Source: CAD feature listing. Evaluate the final solid. Frame: model axes, mm. Round coordinates to 2 decimals unless told otherwise and drop trailing zeros. Write each loop counter-clockwise with the first axis right and the second up, starting at its lowest first coordinate (ties: lowest second). Pieces come first, ordered by that corner, then holes. Notation, with made-up numbers: M -30.75,16 L -11.75,16 A34 cw -11.75,52 Z; hole C -3,-20.75 d6. An arc over 180 degrees is marked long. Answer in a Markdown table with one row per item.
from build123d import *

# Parameters (mm, degrees)
SKETCH1_R           = 4
SKETCH1_R_2         = 2
BOSS_EXTRUDE1_DEPTH = 5
FILLET1_R           = 1


with BuildPart() as part:
    # Sketch1 → Boss-Extrude1 (new body)
    with BuildSketch(Plane.XY):
        Polygon((0, -20), (8, -40), (12, -40), (20, -20), (20, 0), (0, 0), align=None)
        with Locations((9.984598527, -6.114863432)):
            Circle(SKETCH1_R, mode=Mode.SUBTRACT)
        with Locations((9.984598527, -36.114863432)):
            Circle(SKETCH1_R_2, mode=Mode.SUBTRACT)
    extrude(amount=BOSS_EXTRUDE1_DEPTH)

    # Fillet1
    fillet1_edges = [part.edges().sort_by_distance(p)[0] for p in [
        (10, -40, 5),
        (0, 0, 2.5),
        (20, 0, 2.5),
        (20, -20, 2.5),
        (12, -40, 2.5),
        (8, -40, 2.5),
        (0, -20, 2.5),
        (16, -30, 5),
        (20, -10, 5),
        (10, 0, 5),
        (0, -10, 5),
        (10, 0, 0),
        (20, -10, 0),
        (16, -30, 0),
        (4, -30, 5),
        (10, -40, 0),
        (4, -30, 0),
        (0, -10, 0),
    ]]
    fillet(fillet1_edges, radius=FILLET1_R)


solid = part.part
Q1. Section A-A (y = -7). Return loops of the section in (x, z).
Solutions:
| item | result |
|---|---|
| outline | M 0,1 A1 ccw 1,0 L 6.08,0 L 6.08,5 L 1,5 A1 ccw 0,4 Z; M 13.89,0 L 19,0 A1 ccw 20,1 L 20,4 A1 ccw 19,5 L 13.89,5 Z |
Q2. Pull-direction query (X, two-part tool) for faces 1 (the flat face through (0, -10, 2)), 2 (the cylindrical face through (15.88, -29.53, 0.3)), 3 (the cylindrical face through (5.99, -5.94, 2.46)); classes: pulls with the +X half, pulls with the -X half, needs draft (parallel to the pull), parting line crosses it, or undercut.
Solutions:
| item | result |
|---|---|
| face 1 | pulls with the -X half |
| face 2 | pulls with the +X half |
| face 3 | undercut |
Q3. Section B-B (x = 10). Return loops of the section in (y, z).
Solutions:
| item | result |
|---|---|
| outline | M -40,1 A1 ccw -39,0 L -38.11,0 L -38.11,5 L -39,5 A1 ccw -40,4 Z; M -34.11,0 L -10.11,0 L -10.11,5 L -34.11,5 Z; M -2.11,0 L -1,0 A1 ccw 0,1 L 0,4 A1 ccw -1,5 L -2.11,5 Z |
Q4. Material intervals for probe 1 along Y at (x, z) = (10, 1.95); probe 2 along Y at (x, z) = (8.75, 3.3); probe 3 along X at (y, z) = (-9, 1.55), sorted ascending.
Solutions:
| item | result |
|---|---|
| probe 1 | y = -40 to -38.11, -34.11 to -10.11, -2.11 to 0 |
| probe 2 | y = -40 to -37.69, -34.54 to -9.92, -2.31 to 0 |
| probe 3 | x = 0 to 7.21, 12.76 to 20 |
Q5. Section C-C (z = 1.75). Return loops of the section in (x, y).
Solutions:
| item | result |
|---|---|
| outline | M 0,-19.81 A1 ccw 0.07,-20.18 L 7.75,-39.37 A1 ccw 8.68,-40 L 11.32,-40 A1 ccw 12.25,-39.37 L 19.93,-20.18 A1 ccw 20,-19.81 L 20,-1 A1 ccw 19,0 L 1,0 A1 ccw 0,-1 Z; hole C 9.98,-6.11 d8; hole C 9.98,-36.11 d4 |
Q6. Contact query for flat-ended pins moving along their axis: pin 1 Ø6 at (x, y) = (2.5, -32.5) entering from -Z; pin 2 Ø6.5 at (x, y) = (9.98, -6.11) entering from -Z; pin 3 Ø2 at (y, z) = (-23, 2.5) entering from -X. Output: stop coordinate, or through.
Solutions:
| item | result |
|---|---|
| pin 1 | stops at z = 0.05 |
| pin 2 | passes through |
| pin 3 | stops at x = 0.8 |
